Can you work these out from the model? Positions are in its coordinate system, mm. Round coordinates to 2 decimals unless told otherwise and drop trailing zeros. Order: outer loops, then holes, each group sorted by start corner. A loop starts at its lowest first (then second) coordinate and runs counter-clockwise, first axis right, second up. Notation, with made-up numbers: (80.25, 66.5) - (115.25, 66.5) arc R25 ccw to (115.25, 96.5) - close; hole circle Ø3 at (-37, 80). An arc over 180 degrees is marked (long way). Write item = value, one per line.
from build123d import *

# Parameters (mm, degrees)
SKETCH1_W               = 70
SKETCH1_H               = 70
SKETCH1_R               = 1.35
BOSS_EXTRUDE1_DEPTH     = 3.175
FILLET1_R               = 1.5
CUT_EXTRUDE1_DEPTH      = 50.599199842
CUT_EXTRUDE1_DEPTH_BACK = 50.599199842
SKETCH2_W               = 10
SKETCH2_H               = 38
FILLET2_R               = 2
CUT_EXTRUDE2_DEPTH      = 50.599199842
CUT_EXTRUDE2_DEPTH_BACK = 50.599199842
SKETCH3_W               = 22
SKETCH3_H               = 10
SKETCH3_W_2             = 11.75
SKETCH3_H_2             = 8
SKETCH3_W_3             = 5.35
SKETCH3_H_3             = 9
FILLET3_R               = 2


with BuildPart() as part:
    # Sketch1 → Boss-Extrude1 (new body)
    with BuildSketch(Plane.XY):
        Rectangle(SKETCH1_W, SKETCH1_H)
        with Locations((-32.84, 32.82)):
            Circle(SKETCH1_R, mode=Mode.SUBTRACT)
        with Locations((-32.84, -32.84)):
            Circle(SKETCH1_R, mode=Mode.SUBTRACT)
        with Locations((32.82, -32.84)):
            Circle(SKETCH1_R, mode=Mode.SUBTRACT)
        with Locations((32.82, 32.82)):
            Circle(SKETCH1_R, mode=Mode.SUBTRACT)
    extrude(amount=BOSS_EXTRUDE1_DEPTH)

    # Fillet1
    fillet1_edges = [part.edges().sort_by_distance(p)[0] for p in [
        (35, -35, 1.5875),
        (-35, -35, 1.5875),
        (-35, 35, 1.5875),
        (35, 35, 1.5875),
    ]]
    fillet(fillet1_edges, radius=FILLET1_R)

    # Sketch2 → Cut-Extrude1 (cut, two sides: drawn at the far end of the back side and taken through both)
    with BuildSketch(Plane(origin=(0, 0, 0), x_dir=(-1, 0, 0), z_dir=(0, 0, -1)).offset(-CUT_EXTRUDE1_DEPTH_BACK)):
        with Locations((-30, -4.5)):
            Rectangle(SKETCH2_W, SKETCH2_H)
    extrude(amount=CUT_EXTRUDE1_DEPTH + CUT_EXTRUDE1_DEPTH_BACK, mode=Mode.SUBTRACT)

    # Fillet2
    fillet2_edges = [part.edges().sort_by_distance(p)[0] for p in [
        (35, -23.5, 1.5875),
        (25, 14.5, 1.5875),
        (35, 14.5, 1.5875),
        (25, -23.5, 1.5875),
    ]]
    fillet(fillet2_edges, radius=FILLET2_R)

    # Sketch3 → Cut-Extrude2 (cut, two sides: drawn at the far end of the back side and taken through both)
    with BuildSketch(Plane(origin=(0, 0, 0), x_dir=(-1, 0, 0), z_dir=(0, 0, -1)).offset(-CUT_EXTRUDE2_DEPTH_BACK)):
        with Locations((11, -30)):
            Rectangle(SKETCH3_W, SKETCH3_H)
        with Locations((6.125, 31)):
            Rectangle(SKETCH3_W_2, SKETCH3_H_2)
        with Locations((-3.925, -14.5)):
            Rectangle(SKETCH3_W_3, SKETCH3_H_3)
    extrude(amount=CUT_EXTRUDE2_DEPTH + CUT_EXTRUDE2_DEPTH_BACK, mode=Mode.SUBTRACT)

    # Fillet3
    fillet3_edges = [part.edges().sort_by_distance(p)[0] for p in [
        (-22, -35, 1.5875),
        (0, -25, 1.5875),
        (-22, -25, 1.5875),
        (0, -35, 1.5875),
        (-12, 27, 1.5875),
        (-0.25, 35, 1.5875),
        (-12, 35, 1.5875),
        (-0.25, 27, 1.5875),
    ]]
    fillet(fillet3_edges, radius=FILLET3_R)


solid = part.part
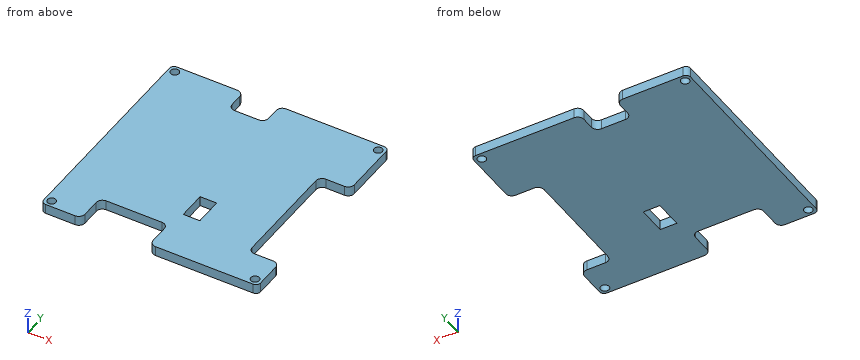
(1) Will this pin go through, and if not, where does the flat tip stop? P1, Ø2, axis at x = 26.5, y = 3, coming from the +Z side.
Computed:
P1 = through
(2) If we section it at B-B (z = 2.5): State how many separate pieces and enclosed holes the cut face has, plus the area to 3 significant figures.
Computed:
separate_pieces = 1
enclosed_holes = 5
area = 4,130 mm^2
(3) If we section it at C-C (y = 4.5): Write out the boundary of the cut face in (x, z) (3 decimals), plus the area to 4 significant figures.
Computed:
outline = (-35, 0) - (25, 0) - (25, 3.175) - (-35, 3.175) - close
area = 190.5 mm^2
(4) If we section it at A-A (x = 30.5): Write out the boundary of the cut face in (y, z) (3 decimals), plus the area to 3 significant figures.
Computed:
outline = (-35, 0) - (-23.5, 0) - (-23.5, 3.175) - (-35, 3.175) - close; (14.5, 0) - (35, 0) - (35, 3.175) - (14.5, 3.175) - close
area = 102 mm^2
(5) If I drill on line 1 (Y direction, x = -32.84, z = 1.2); line 2 (Y direction, x = 32.82, z = 2.4); line 3 (X direction, y = -30.5, z = 1), over which ranges is the centre line in solid material (lowest first)? Write a range as from..to.
Computed:
line_1 = -35..-34.19, -31.49..31.47, 34.17..35
line_2 = -35..-34.19, -31.49..-23.5, 14.5..31.47, 34.17..35
line_3 = -35..-22, 0..35
